Build history of the part. All positions in model axes, mm. Face numbers are marked on the shaded views. A direction names the side the tool comes from. Give positions to 0.01 mm unless a question says otherwise; leave off trailing zeros. Order: outer loops, then holes, each group sorted by start corner. A loop starts at its lowest first (then second) coordinate and runs counter-clockwise, first axis right, second up. Notation, with made-up numbers: (39, 80) -> (94, 80) arc R22 cw to (94, 108) -> close; hole circle Ø6 at (66.5, 52.25). An arc over 180 degrees is marked (long way). Write item = value, one per line. Start each with the question number.
from build123d import *

# Parameters (mm, degrees)
BOSS_EXTRUDE1_DEPTH = 69.85
FILLET1_R           = 5.08
FILLET3_R           = 2.54
CUT_EXTRUDE1_REACH  = 93.204
FILLET2_R           = 7.62
FILLET4_R           = 12.7


with BuildPart() as part:
    # Sketch1 → Boss-Extrude1 (new body)
    with BuildSketch(Plane.XY):
        Polygon((-76.2, 6.735192091), (-27.998371742, 54.936820349), (-24.630775696, 51.569224304), (-71.4375, 4.7625), (-4.7625, 4.7625), (-4.7625, 12.7), (0, 12.7), (0, 6.630240755), (0, 0), (-76.2, 0), align=None)
    extrude(amount=BOSS_EXTRUDE1_DEPTH)

    # Fillet1
    # the kernel refuses this fillet: 5.08 mm, written as the material it adds along each edge
    with BuildSketch(Plane(origin=(-4.7625, 4.7625, 0), x_dir=(0, 1, 0), z_dir=(0, 0, 1))) as fillet1_piece_1:
        with BuildLine():
            CenterArc((FILLET1_R, FILLET1_R), FILLET1_R, 180, 90)
            Line((0, FILLET1_R), (0, 0))
            Line((0, 0), (FILLET1_R, 0))
        make_face()
    extrude(amount=69.85)
    # the kernel refuses this fillet: 5.08 mm, written as the material it takes off along each edge
    with BuildSketch(Plane(origin=(-76.2, 0, -12.7), x_dir=(0, 1, 0), z_dir=(0, 0, 1)), Plane(origin=(0, 0, -12.7), x_dir=(-1, 0, 0), z_dir=(0, 0, 1))) as fillet1_2_piece_1:
        with BuildLine():
            CenterArc((FILLET1_R, -FILLET1_R), FILLET1_R, 90, 90)
            Line((0, -FILLET1_R), (0, 0))
            Line((0, 0), (FILLET1_R, 0))
        make_face()
    extrude(amount=95.25, mode=Mode.SUBTRACT)
    with BuildSketch(Plane(origin=(-76.2, 6.735192091, -5.260512242), x_dir=(0.7071067811865465, 0.7071067811865486, 0), z_dir=(0, 0, 1))) as fillet1_2_piece_2:
        with BuildLine():
            CenterArc((FILLET1_R * 0.414213562373, -FILLET1_R), FILLET1_R, 90, 45)
            Line((-FILLET1_R * 0.292893218813, -FILLET1_R * 0.292893218813), (0, 0))
            Line((0, 0), (FILLET1_R * 0.414213562373, 0))
        make_face()
    extrude(amount=80.371024484, mode=Mode.SUBTRACT)

    # Fillet3
    fillet3_edges = [part.edges().sort_by_distance(p)[0] for p in [
        (-71.4375, 4.7625, 34.925),
    ]]
    fillet(fillet3_edges, radius=FILLET3_R)

    # Sketch2 → Cut-Extrude1 (cut, up to next)
    with BuildSketch(Plane(origin=(-41.467596045, 41.467596045, 0), x_dir=(0, 0, 1), z_dir=(-0.7071067811865489, 0.7071067811865462, 0)), mode=Mode.PRIVATE) as cut_extrude1_sk1:
        Polygon((15.875, 19.048359685), (0, -41.014242187), (0, 19.048359685), align=None)
    cut_extrude1_tool1 = extrude(cut_extrude1_sk1.sketch, amount=-CUT_EXTRUDE1_REACH, mode=Mode.PRIVATE) & part.part
    # Sketch2 → Cut-Extrude1 (cut, up to next)
    with BuildSketch(Plane(origin=(-41.467596045, 41.467596045, 0), x_dir=(0, 0, 1), z_dir=(-0.7071067811865489, 0.7071067811865462, 0)), mode=Mode.PRIVATE) as cut_extrude1_sk2:
        Polygon((69.85, 19.048359685), (53.975, 19.048359685), (69.85, -41.014242187), align=None)
    cut_extrude1_tool2 = extrude(cut_extrude1_sk2.sketch, amount=-CUT_EXTRUDE1_REACH, mode=Mode.PRIVATE) & part.part
    add(cut_extrude1_tool1.solids().sort_by_distance((-42.155263, 40.779929, 5.291667))[0], mode=Mode.SUBTRACT)
    add(cut_extrude1_tool2.solids().sort_by_distance((-42.155263, 40.779929, 64.558333))[0], mode=Mode.SUBTRACT)

    # Fillet2
    fillet2_edges = [part.edges().sort_by_distance(p)[0] for p in [
        (-2.38125, 12.7, 0),
        (-2.38125, 12.7, 69.85),
        (-26.314573719, 53.253022326, 53.975),
        (-26.314573719, 53.253022326, 15.875),
    ]]
    fillet(fillet2_edges, radius=FILLET2_R)

    # Fillet4
    fillet4_edges = [part.edges().sort_by_distance(p)[0] for p in [
        (-68.785246798, 10.782349247, 0),
        (-68.785246798, 10.782349247, 69.85),
    ]]
    fillet(fillet4_edges, radius=FILLET4_R)


solid = part.part
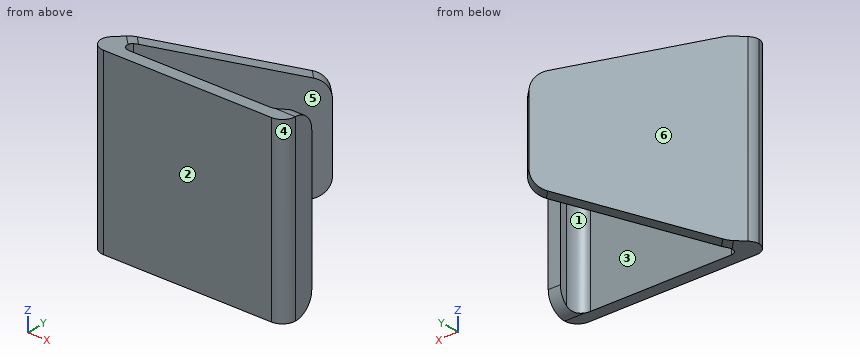
(1) Cut at D-D, the plane y = 45. Give the cut face in (x, z).
(2) Cut at C-C, the plane x = -63. Give the cut face in (y, z).
(3) Cut at B-B, the plane z = 34.5. Give the cut face in (x, y).
(4) Wall check: line 1 (Y direction, x = -10, z = 62.5); line 2 (Y direction, x = -64, z = 52.5); line 3 (X direction, y = 6, z = 23). Give the ranges that are in metal, low to high. Write a range as [from, to].
(5) 3-axis set-ups, long thin cutter, end or side, ignore diameter. For the marked faces 1, 2 and 3: which of +Z, -Z, +X, -X, +Y, -Y reach the whole face in a straight line?
(6) Mould opens along Y. For the marked faces 4, 5 and 6 say: released by +Y, released by -Y, zero draft, split by the parting line, or undercut.
(7) Flat gauge pins, fed straight in: P1, Ø10, axis at x = -46.5, z = 41.5, coming from the +Y side; P2, Ø8, axis at x = -43, y = 33.5, coming from the +Z side; P3, Ø2, axis at x = -33, z = 24, coming from the -Y side; P4, Ø12, axis at x = -39.5, y = 39.5, coming from the +Z side. Where does each tip first touch, or does it go through?
(8) Cut at A-A, the plane x = -45. Give the cut face in (y, z).
Results:
q1.outline = (-37.94, 12.16) -> (-31.2, 13.42) -> (-31.2, 56.43) -> (-37.94, 57.69) -> close
q2.outline = (0, 0) -> (4.76, 0) -> (4.76, 69.85) -> (0, 69.85) -> close; (13.2, 1.53) -> (19.94, 2.79) -> (19.94, 67.06) -> (13.2, 68.32) -> close
q3.outline = (-76.2, 4.86) arc R5.08 ccw to (-71.12, 0) -> (-5.08, 0) arc R5.08 ccw to (0, 5.08) -> (0, 12.7) -> (-4.76, 12.7) -> (-4.76, 9.84) arc R5.08 cw to (-9.84, 4.76) -> (-65.31, 4.76) arc R2.54 cw to (-67.1, 9.1) -> (-24.63, 51.57) -> (-28, 54.94) -> (-74.71, 8.22) arc R5.08 ccw to start
q4.line_1 = [0, 4.76]
q4.line_2 = [0, 4.76], [12.2, 18.94]
q4.line_3 = [-76.01, -67.49], [-6.52, 0]
q5.face_1 = +Z, -Z, +Y
q5.face_2 = +Z, -Z, +X, -X, -Y
q5.face_3 = +Z, -Z
q6.face_4 = released by -Y
q6.face_5 = undercut
q6.face_6 = released by +Y
q7.P1 = 41.44
q7.P2 = 61.84
q7.P3 = 0
q7.P4 = 60.6
q8.outline = (0, 0) -> (4.76, 0) -> (4.76, 69.85) -> (0, 69.85) -> close; (31.2, 8.26) -> (37.94, 9.52) -> (37.94, 60.33) -> (31.2, 61.59) -> close
